Build history of the part. All positions in model axes, mm. Face numbers are marked on the shaded views. A direction names the side the tool comes from. Give positions to 0.01 mm unless a question says otherwise; leave off trailing zeros. Write each loop counter-clockwise with the first axis right and the second up, starting at its lowest first coordinate (ties: lowest second). Pieces come first, ordered by that corner, then holes.
from build123d import *

# Parameters (mm, degrees)
F1_DEPTH = 400
F2_R     = 25
F3_DEPTH = 400
F5_DEPTH = 1500


with BuildPart() as f1:
    # F0 (on Front) → F1 (new body, symmetric)
    with BuildSketch(Plane.XZ):
        Polygon((750, 0), (-750, 0), (-750, -600), (-500, -1000), (500, -1000), (750, -600), align=None)
    extrude(amount=F1_DEPTH, both=True)

    # F2 (on Front) → F3 (join, symmetric)
    with BuildSketch(Plane.XZ):
        with BuildLine():
            Line((-32.921014, 337.789664), (-455.401369, -84.690691))
            ThreePointArc((-455.401369, -84.690691), (-460.755214, -158.795816), (-386.474404, -157.185082))
            Line((-386.474404, -157.185082), (-79.289322, 150))
            Line((-79.289322, 150), (0, 150))
            Line((0, 150), (79.289322, 150))
            Line((79.289322, 150), (386.474404, -157.185082))
            ThreePointArc((386.474404, -157.185082), (460.755214, -158.795816), (455.401369, -84.690691))
            Line((455.401369, -84.690691), (32.921014, 337.789664))
            ThreePointArc((32.921014, 337.789664), (0, 351.28622), (-32.921014, 337.789664))
        make_face()
        with Locations((0, 300)):
            Circle(F2_R, mode=Mode.SUBTRACT)
    extrude(amount=F3_DEPTH, both=True)

    # F4 (on face) → F5 (cut)
    with BuildSketch(Plane.YZ.offset(750)):
        Polygon((200, 500), (-200, 500), (-200, 0), (-200, -200), (200, -200), (200, 0), align=None)
    extrude(amount=-F5_DEPTH, mode=Mode.SUBTRACT)


solid = f1.part
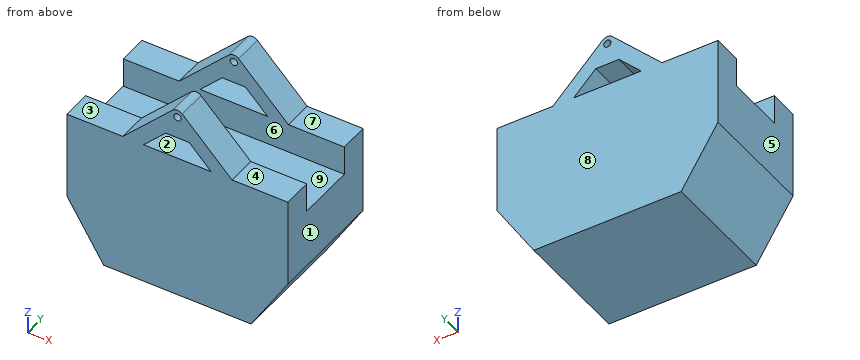
1. Drill centre lines: line 1 along Y through (x, z) = (-350, -158); line 2 along Z through (x, y) = (-72, 233); line 3 along X through (y, z) = (-324, 300). Where is each one in solid material? Low to high.
2. Mould opens along Y. For the marked faces 6, 7, 8 and 9 say: pulls with the +Y half, pulls with the -Y half, needs draft (parallel to the pull), parting line crosses it, or undercut.
3. 3-axis set-ups, long thin cutter, end or side, ignore diameter. For the marked faces 1, 2, 3, 4 and 5: which of +Z, -Z, +X, -X, +Y, -Y reach the whole face in a straight line?
4. Saw through at A-A on y = 275. Give the cut face in (x, z), plus the area to 3 significant figures.
5. Saw through at B-B on x = 0. Give the cut face in (y, z).
6. Saw through at D-D on y = -164. Give the cut face in (x, z), plus the area to 3 significant figures.
7. Saw through at C-C on z = 300. Give the cut face in (x, y).
8. Drop a flat-ended pin along its axis: pin 1 (5 mm diameter, centred on x = -233.5, y = 179.5, fed in from +Z). Give the stop position or say it passes through.
Outcome:
1. line 1: y = -400 to -200, 200 to 400
1. line 2: z = -1000 to 0, 150 to 298.71
1. line 3: x = -70.71 to -25, 25 to 70.71
2. face 6: undercut
2. face 7: needs draft
2. face 8: pulls with the +Y half
2. face 9: undercut
3. face 1: +Z, -Z, +X, +Y, -Y
3. face 2: +Y, -Y
3. face 3: +Z, -X, +Y, -Y
3. face 4: +Z, +X, +Y, -Y
3. face 5: +Z, -Z, -X, +Y, -Y
4. outline: (-750, -600) - (-500, -1000) - (500, -1000) - (750, -600) - (750, 0) - (370.71, 0) - (32.92, 337.79) arc R46.9 ccw to (-32.92, 337.79) - (-370.71, 0) - (-750, 0) - close; hole (-229.29, 0) - (229.29, 0) - (79.29, 150) - (-79.29, 150) - close; hole circle Ø50 at (0, 300)
4. area: 1,490,000 mm2
5. outline: (-400, -1000) - (400, -1000) - (400, 0) - (200, 0) - (200, -200) - (-200, -200) - (-200, 0) - (-400, 0) - close; (-400, 150) - (-200, 150) - (-200, 275) - (-400, 275) - close; (-400, 325) - (-200, 325) - (-200, 351.29) - (-400, 351.29) - close; (200, 150) - (400, 150) - (400, 275) - (200, 275) - close; (200, 325) - (400, 325) - (400, 351.29) - (200, 351.29) - close
6. outline: (-750, -600) - (-500, -1000) - (500, -1000) - (750, -600) - (750, -200) - (-750, -200) - close
6. area: 1,100,000 mm2
7. outline: (-70.71, -400) - (-25, -400) - (-25, -200) - (-70.71, -200) - close; (-70.71, 200) - (-25, 200) - (-25, 400) - (-70.71, 400) - close; (25, -400) - (70.71, -400) - (70.71, -200) - (25, -200) - close; (25, 200) - (70.71, 200) - (70.71, 400) - (25, 400) - close
8. pin 1: stops at z = -200
